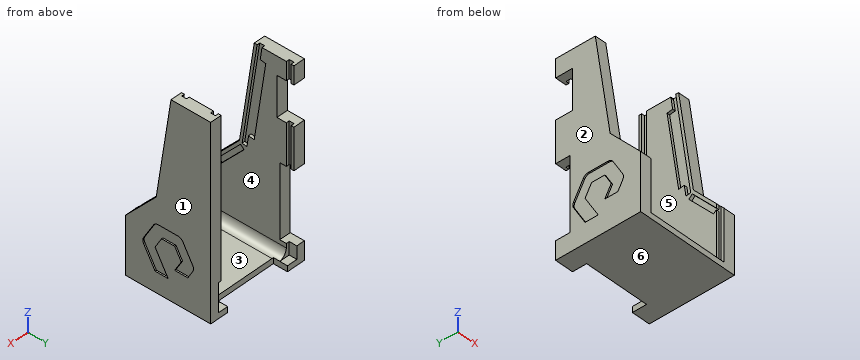
from build123d import *

# Parameters (mm, degrees)
F1_DEPTH     = 18
F2_W         = 30
F2_H         = 80
F3_DEPTH     = 14
F4_W         = 5
F4_H         = 25.6
F4_W_2       = 6
F4_H_2       = 14
F5_DEPTH     = 25
F6_W         = 5
F6_H         = 5
F7_DEPTH     = 11.5
F8_W         = 10
F8_H         = 10
F9_DEPTH     = 15.1
F10_W        = 1.7
F10_H        = 17.78
F10_H_2      = 10
F11_DEPTH    = 15.1
F13_DEPTH    = 15.1
F15_DEPTH    = 15
F17_DEPTH    = 0.5
F19_DEPTH    = 0.5
F20_T4_DEPTH = 32.1
F20_T9_DEPTH = 32.1
F21_T4_DEPTH = 32.1
F21_T9_DEPTH = 24.6


# Not quite as in the source:
# - a fillet or chamfer that OpenCascade refuses, or shapes differently, is made with other operations: its cross-section is extruded or revolved along the edge and cut away or added


with BuildPart() as f1:
    # F0 (on Right) → F1 (new body, symmetric)
    with BuildSketch(Plane.YZ):
        Polygon((-30, 0), (0, 0), (0, 67), (-14, 67), (-19.2224497622, 31.8255828978), (-30, 20), align=None)
    extrude(amount=F1_DEPTH, both=True)

    # F2 (on Right) → F3 (cut, symmetric)
    with BuildSketch(Plane.YZ):
        with Locations((-15, 42)):
            Rectangle(F2_W, F2_H)
    extrude(amount=F3_DEPTH, both=True, mode=Mode.SUBTRACT)

    # F4 (on Right) → F5 (cut)
    with BuildSketch(Plane.YZ):
        with Locations((-2.5, 19.3)):
            Rectangle(F4_W, F4_H)
        with Locations((-3, 53.6)):
            Rectangle(F4_W_2, F4_H_2)
    extrude(amount=-F5_DEPTH, mode=Mode.SUBTRACT)

    # F6 (on Right) → F7 (cut, symmetric)
    with BuildSketch(Plane.YZ):
        with Locations((-2.5, 2.5)):
            Rectangle(F6_W, F6_H)
    extrude(amount=F7_DEPTH, both=True, mode=Mode.SUBTRACT)

    # F8 (on Right) → F9 (cut, symmetric)
    with BuildSketch(Plane.YZ):
        Polygon((-2.7, 67), (-2.7, 2), (-1, 2), (-1, 12), (-1, 67), align=None)
        with Locations((4, 7)):
            Rectangle(F8_W, F8_H)
    extrude(amount=F9_DEPTH, both=True, mode=Mode.SUBTRACT)

    # F10 (on Right) → F11 (cut, symmetric)
    with BuildSketch(Plane.YZ):
        with Locations((-28.15, 10.89)):
            Rectangle(F10_W, F10_H)
        with Locations((-28.15, 24.78)):
            Rectangle(F10_W, F10_H_2)
    extrude(amount=F11_DEPTH, both=True, mode=Mode.SUBTRACT)

    # F12 (on Right) → F13 (cut, symmetric)
    with BuildSketch(Plane.YZ):
        Polygon((-17.5946665501, 29.6033232788), (-18.851134733, 30.7484379915), (-27.5769088442, 21.1741504379), (-26.3204406613, 20.0290357252), align=None)
    extrude(amount=F13_DEPTH, both=True, mode=Mode.SUBTRACT)

    # F14 (on Right) → F15 (cut, symmetric)
    with BuildSketch(Plane.YZ):
        Polygon((-11.9167287085, 62.6468424419), (-11.3292765417, 66.6034697875), (-13.0108431636, 66.8531369583), (-18.2705961384, 31.4274740197), (-16.5890295165, 31.1778068488), (-16.0015773498, 35.1344341944), align=None)
        Polygon((-13.0108431636, 66.8531369583), (-11.3292765417, 66.6034697875), (-9.8606461249, 76.4950381514), (-11.5422127468, 76.7447053223), align=None)
        Polygon((-9.9384150357, 62.3531163585), (-11.9167287085, 62.6468424419), (-16.0015773498, 35.1344341944), (-14.023263677, 34.840708111), align=None)
    extrude(amount=F15_DEPTH, both=True, mode=Mode.SUBTRACT)

    # F16 (on face) → F17 (cut)
    with BuildSketch(Plane.YZ.offset(18)):
        with BuildLine():
            Line((-19.6188021535, 7), (-15, 7))
            Line((-15, 7), (-17.3094010768, 11))
            Line((-17.3094010768, 11), (-19.6188021535, 15))
            Line((-19.6188021535, 15), (-17.3094010768, 19))
            Line((-17.3094010768, 19), (-12.6905989232, 19))
            Line((-12.6905989232, 19), (-10.3811978465, 15))
            Line((-10.3811978465, 15), (-12.6905989232, 11))
            Line((-12.6905989232, 11), (-8.0717967697, 11))
            Line((-8.0717967697, 11), (-6.3397459622, 14))
            ThreePointArc((-6.3397459622, 14), (-6.0717967697, 15), (-6.3397459622, 16))
            Line((-6.3397459622, 16), (-9.8038475773, 22))
            ThreePointArc((-9.8038475773, 22), (-10.5358983849, 22.7320508076), (-11.5358983849, 23))
            Line((-11.5358983849, 23), (-18.4641016151, 23))
            ThreePointArc((-18.4641016151, 23), (-19.4641016151, 22.7320508076), (-20.1961524227, 22))
            Line((-20.1961524227, 22), (-23.6602540378, 16))
            ThreePointArc((-23.6602540378, 16), (-23.9282032303, 15), (-23.6602540378, 14))
            Line((-23.6602540378, 14), (-19.6188021535, 7))
        make_face()
    extrude(amount=-F17_DEPTH, mode=Mode.SUBTRACT)

    # F18 (on face) → F19 (cut)
    with BuildSketch(Plane(origin=(-18, 0, 0), x_dir=(0, -1, 0), z_dir=(-1, 0, 0))):
        with BuildLine():
            Line((18.4641016151, 23), (11.5358983849, 23))
            ThreePointArc((11.5358983849, 23), (10.5358983849, 22.7320508076), (9.8038475773, 22))
            Line((9.8038475773, 22), (6.3397459622, 16))
            ThreePointArc((6.3397459622, 16), (6.0717967697, 15), (6.3397459622, 14))
            Line((6.3397459622, 14), (10.3811978465, 7))
            Line((10.3811978465, 7), (15, 7))
            Line((15, 7), (12.6905989232, 11))
            Line((12.6905989232, 11), (10.3811978465, 15))
            Line((10.3811978465, 15), (12.6905989232, 19))
            Line((12.6905989232, 19), (17.3094010768, 19))
            Line((17.3094010768, 19), (19.6188021535, 15))
            Line((19.6188021535, 15), (17.3094010768, 11))
            Line((17.3094010768, 11), (21.9282032303, 11))
            Line((21.9282032303, 11), (23.6602540378, 14))
            ThreePointArc((23.6602540378, 14), (23.9282032303, 15), (23.6602540378, 16))
            Line((23.6602540378, 16), (20.1961524227, 22))
            ThreePointArc((20.1961524227, 22), (19.4641016151, 22.7320508076), (18.4641016151, 23))
        make_face()
    extrude(amount=-F19_DEPTH, mode=Mode.SUBTRACT)

    # F20: fillet of radius 3 on 1 edges, made by hand


with BuildPart() as f20_tool2:
    # F20_s3 → F20_t4 (new body)
    with BuildSketch(Plane.XZ.offset(27.3)):
        with BuildLine():
            ThreePointArc((-14, 5), (-13.1213203436, 2.8786796564), (-11, 2))
            Line((-11, 2), (-14, 2))
            Line((-14, 2), (-14, 5))
        make_face()
    extrude(amount=-F20_T4_DEPTH)

    split(bisect_by=Plane.XZ.offset(5), keep=Keep.TOP)


with BuildPart() as f1_1:
    add(f1.part)

    # F20_t1: union F20_tool2
    add(f20_tool2.part)


with BuildPart() as f20_tool7:
    # F20_s8 → F20_t9 (new body)
    with BuildSketch(Plane.XZ.offset(34.8)):
        with BuildLine():
            ThreePointArc((-14, 5), (-13.1213203436, 2.8786796564), (-11, 2))
            Line((-11, 2), (-14, 2))
            Line((-14, 2), (-14, 5))
        make_face()
    extrude(amount=-F20_T9_DEPTH)

    split(bisect_by=Plane.YZ.offset(-11.5), keep=Keep.BOTTOM)

    split(bisect_by=Plane.XZ.offset(5), keep=Keep.BOTTOM)


with BuildPart() as f1_2:
    add(f1_1.part)

    # F20_t6: union F20_tool7
    add(f20_tool7.part)

    # F21: fillet of radius 3 on 1 edges, made by hand


with BuildPart() as f21_tool2:
    # F21_s3 → F21_t4 (new body)
    with BuildSketch(Plane.XZ.offset(27.3)):
        with BuildLine():
            ThreePointArc((11, 2), (13.1213203436, 2.8786796564), (14, 5))
            Line((14, 5), (14, 2))
            Line((14, 2), (11, 2))
        make_face()
    extrude(amount=-F21_T4_DEPTH)

    split(bisect_by=Plane.XZ.offset(5), keep=Keep.TOP)


with BuildPart() as f1_3:
    add(f1_2.part)

    # F21_t1: union F21_tool2
    add(f21_tool2.part)


with BuildPart() as f21_tool7:
    # F21_s8 → F21_t9 (new body)
    with BuildSketch(Plane.XZ.offset(27.3)):
        with BuildLine():
            ThreePointArc((11, 2), (13.1213203436, 2.8786796564), (14, 5))
            Line((14, 5), (14, 2))
            Line((14, 2), (11, 2))
        make_face()
    extrude(amount=-F21_T9_DEPTH)

    split(bisect_by=Plane.YZ.offset(11.5), keep=Keep.TOP)


with BuildPart() as f1_4:
    add(f1_3.part)

    # F21_t6: union F21_tool7
    add(f21_tool7.part)


solid = f1_4.part
Read the model definition and answer for the solid it produces. Units are mm, in the model's axes. Face numbers are marked on the shaded views. A direction names the side the tool comes from. Round coordinates to 2 decimals unless told otherwise and drop trailing zeros. Write each loop counter-clockwise with the first axis right and the second up, starting at its lowest first coordinate (ties: lowest second). Pieces come first, ordered by that corner, then holes.
Q1. Flat-ended cylindrical pins translate along their axes: P1, Ø0.6, axis at x = 17.5, y = -14, coming from the -Z side; P2, Ø1.1, axis at x = -12.5, z = 3.5, coming from the +Y side; P3, Ø1.5, axis at y = -22, z = 15.5, coming from the +X side; P4, Ø4.5, axis at x = -16, z = 16.5, coming from the +Y side. Find the tip coordinate at first contact, or state that the pin passes through.
Values:
P1: stops at z = 0
P2: passes through
P3: stops at x = 17.5
P4: stops at y = -5
Q2. Find section B-B on z = 26. Determine the outline of the cut face in (x, y), and give its area (3 significant figures).
Values:
outline: (-18, -24.53) - (-14, -24.53) - (-14, -23.18) - (-15.1, -23.18) - (-15.1, -20.88) - (-14, -20.88) - (-14, -5) - (-18, -5) - close; (14, -24.53) - (18, -24.53) - (18, 0) - (14, 0) - (14, -1) - (15.1, -1) - (15.1, -2.7) - (14, -2.7) - (14, -20.88) - (15.1, -20.88) - (15.1, -23.18) - (14, -23.18) - close
area: 169 mm2
Q3. Straight lines are drawn through the part: line 1 (X direction, y = -22, z = 27.5); line 2 (X direction, y = -12, z = 22.5); line 3 (Z direction, x = -3.5, y = -21). For each, find the intervals that lie inside material, in ascending order.
Values:
line 1: x = -18 to -14, 14 to 18
line 2: x = -17.5 to -14, 14 to 17.5
line 3: z = 0 to 2
Q4. The mould has two halves that part along X. Classify the marked faces 1, 2, 3 and 4: released by +X, released by -X, zero draft, split by the parting line, or undercut.
Values:
face 1: released by +X
face 2: released by -X
face 3: undercut
face 4: undercut
Q5. Find section A-A on y = -3.5. Determine the outline of the cut face in (x, z).
Values:
outline: (-18, 0) - (-11.5, 0) - (-11.5, 2.04) arc R3 cw to (-14, 5) - (-14, 6.5) - (-18, 6.5) - close; (-18, 32.1) - (-14, 32.1) - (-14, 46.6) - (-18, 46.6) - close; (-18, 60.6) - (-14, 60.6) - (-14, 67) - (-18, 67) - close; (11.5, 0) - (18, 0) - (18, 67) - (14, 67) - (14, 5) arc R3 cw to (11.5, 2.04) - close
Q6. A tool of negligible diameter and unlimited length cuts with its end or side. For the marked faces 5 and 6, from which of +Z, -Z, +X, -X, +Y, -Y can it reach the whole face along a straight path? Write none if from no direction.
Values:
face 5: +Z, +Y, -Y
face 6: -Z, +X, -X, +Y, -Y
Q7. Find section C-C on z = 42. Determine the outline of the cut face in (x, y).
Values:
outline: (-18, -17.71) - (-14, -17.71) - (-14, -16.7) - (-15, -16.7) - (-15, -12.96) - (-14, -12.96) - (-14, -2.7) - (-15.1, -2.7) - (-15.1, -1) - (-14, -1) - (-14, 0) - (-18, 0) - close; (14, -17.71) - (18, -17.71) - (18, 0) - (14, 0) - (14, -1) - (15.1, -1) - (15.1, -2.7) - (14, -2.7) - (14, -12.96) - (15, -12.96) - (15, -16.7) - (14, -16.7) - close
Q8. Find section D-D on x = 5. Determine the outline of the cut face in (y, z), and give its area (3 significant figures).
Values:
outline: (-30, 0) - (-5, 0) - (-5, 2) - (-30, 2) - close
area: 50.0 mm2
